Here's how the part is built. I have some questions about the finished solid (model axes, mm). Face numbers are marked on the shaded views. A direction names the side the tool comes from. Coordinates: 2 decimals unless noted, no trailing zeros. Write each loop counter-clockwise with the first axis right and the second up, starting at its lowest first coordinate (ties: lowest second). Pieces come first, ordered by that corner, then holes.
```python
from build123d import *

# Parameters (mm, degrees)
SKETCH1_W           = 84.836
SKETCH1_H           = 69.342
BASE_FLANGE1_DEPTH  = 4.826
SKETCH6_R           = 2.54
CUT_EXTRUDE1_DEPTH  = 10
FILLET1_R           = 2.6
SKETCH7_W           = 18.5
SKETCH7_H           = 10
SKETCH7_W_2         = 39.8249902
SKETCH7_H_2         = 5
CUT_EXTRUDE2_DEPTH  = 4.826
FILLET2_R           = 2.4
FILLET3_R           = 1.6
SKETCH11_W          = 4.445
SKETCH11_H          = 18.2239968
SKETCH11_H_2        = 48.82401137
SKETCH11_W_2        = 50.8
SKETCH11_H_3        = 4.445
BOSS_EXTRUDE1_DEPTH = 24.638


# Sheet-metal steps are written as plain solids
with BuildPart() as part:
    # Sketch1 → Base-Flange1 (new body)
    with BuildSketch(Plane.XY):
        Rectangle(SKETCH1_W, SKETCH1_H)
    extrude(amount=-BASE_FLANGE1_DEPTH)

    # Sketch6 → Cut-Extrude1 (cut)
    with BuildSketch(Plane.XY):
        with Locations((-37.465, 29.718)):
            Circle(SKETCH6_R)
        with Locations(Location((-37.465, -29.718, 0), (0, 0, 180))):
            Circle(SKETCH6_R)
        with Locations((37.465, -29.718)):
            Circle(SKETCH6_R)
        with Locations(Location((37.465, 29.718, 0), (0, 0, 180))):
            Circle(SKETCH6_R)
    extrude(amount=-CUT_EXTRUDE1_DEPTH, mode=Mode.SUBTRACT)

    # Fillet1
    fillet1_edges = [part.edges().sort_by_distance(p)[0] for p in [
        (-42.418, 34.671, -2.413),
        (42.418, 34.671, -2.413),
        (42.418, -34.671, -2.413),
        (-42.418, -34.671, -2.413),
    ]]
    fillet(fillet1_edges, radius=FILLET1_R)

    # Sketch7 → Cut-Extrude2 (cut)
    with BuildSketch(Plane.XY):
        with Locations((-33.168, 18.7119922)):
            Rectangle(SKETCH7_W, SKETCH7_H)
        Polygon((-42.418, -4.5120046), (-27.432, -4.5120046), (-27.432, -26.512012), (-35.052, -26.512012), (-35.052, -17.5120046), (-42.418, -17.5120046), align=None)
        with Locations((7.7044931, 24.3120114)):
            Rectangle(SKETCH7_W_2, SKETCH7_H_2)
        Polygon((-14.2080054, -21.81200997), (-14.2080054, -1.41199997), (-23.2080054, -1.41199997), (-23.2080054, -26.81199997), (27.6169882, -26.81199997), (27.6169882, -21.81200997), align=None)
        Polygon((24.638, 3.195999958), (-11.43, 3.195999958), (-11.43, 15.895999958), (29.21, 15.895999958), (29.21, 3.195999958), (29.21, -6.804000042), (24.638, -6.804000042), align=None)
    extrude(amount=-CUT_EXTRUDE2_DEPTH, mode=Mode.SUBTRACT)

    # Fillet2
    fillet2_edges = [part.edges().sort_by_distance(p)[0] for p in [
        (-12.208002, 21.8120114, -2.413),
        (-12.208002, 26.8120114, -2.413),
        (27.6169882, 26.8120114, -2.413),
        (27.6169882, 21.8120114, -2.413),
        (27.6169882, -21.81200997, -2.413),
        (27.6169882, -26.81199997, -2.413),
        (-23.2080054, -26.81199997, -2.413),
        (-14.2080054, -21.81200997, -2.413),
        (24.638, 3.195999958, -2.413),
        (-27.432, -26.512012, -2.413),
        (-35.052, -26.512012, -2.413),
    ]]
    fillet(fillet2_edges, radius=FILLET2_R)

    # Fillet3
    fillet3_edges = [part.edges().sort_by_distance(p)[0] for p in [
        (-23.2080054, -1.41199997, -2.413),
        (-14.2080054, -1.41199997, -2.413),
        (24.638, -6.804000042, -2.413),
        (-11.43, 3.195999958, -2.413),
        (-11.43, 15.895999958, -2.413),
        (29.21, 15.895999958, -2.413),
        (29.21, -6.804000042, -2.413),
        (-23.918, 23.7119922, -2.413),
        (-23.918, 13.7119922, -2.413),
        (-27.432, -4.5120046, -2.413),
    ]]
    fillet(fillet3_edges, radius=FILLET3_R)

    # Sketch11 → Boss-Extrude1 (add)
    with BuildSketch(Plane(origin=(0, 0, -4.826), x_dir=(-1, 0, 0), z_dir=(0, 0, -1))):
        with Locations((40.1955, 4.5999938)):
            Rectangle(SKETCH11_W, SKETCH11_H)
        with Locations((-40.1955, 5.715e-06)):
            Rectangle(SKETCH11_W, SKETCH11_H_2)
        with Locations((-0.463533105, -32.4485)):
            Rectangle(SKETCH11_W_2, SKETCH11_H_3)
        with Locations((-0.463533105, 32.4485)):
            Rectangle(SKETCH11_W_2, SKETCH11_H_3)
    extrude(amount=BOSS_EXTRUDE1_DEPTH)


solid = part.part
```
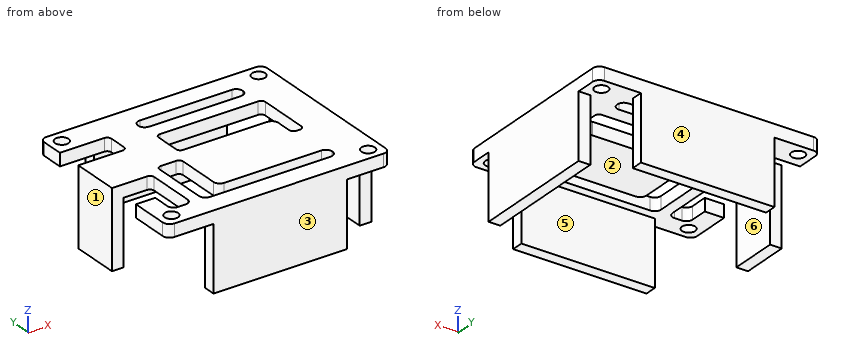
1) I need wall thicknesses on probe 1 along Y at (x, z) = (-6, -0.75); probe 2 along X at (y, z) = (10, -7.25); probe 3 along Y at (x, z) = (-12.5, -25.25). Which ranges of each line are inside material? Lowest first, please.
Values follow:
probe 1: y = -34.67 to -26.81, -21.81 to 3.2, 15.9 to 21.81, 26.81 to 34.67
probe 2: x = -42.42 to -37.97, 37.97 to 42.42
probe 3: y = -34.67 to -30.23, 30.23 to 34.67
2) Imagine slicing it at A-A on z = -12. Please give me the cut outline in (x, y).
Values follow:
outline: (-42.42, -4.51) - (-37.97, -4.51) - (-37.97, 13.71) - (-42.42, 13.71) - close; (-24.94, -34.67) - (25.86, -34.67) - (25.86, -30.23) - (-24.94, -30.23) - close; (-24.94, 30.23) - (25.86, 30.23) - (25.86, 34.67) - (-24.94, 34.67) - close; (37.97, -24.41) - (42.42, -24.41) - (42.42, 24.41) - (37.97, 24.41) - close
3) We'd pull the mould along X, two halves only. Please class the marked faces 1, 2 and 3: pulls with the +X half, pulls with the -X half, needs draft (parallel to the pull), parting line crosses it, or undercut.
Values follow:
face 1: pulls with the -X half
face 2: undercut
face 3: needs draft
4) Will these pins go through, and if not, where does the flat tip stop? pin 1 (4 mm diameter, centred on x = 26.5, z = -9.5, fed in from +Y); pin 2 (1.3 mm diameter, centred on x = 41, z = -18.5, fed in from +Y); pin 3 (1 mm diameter, centred on x = 28, y = -3, fed in from -Z); pin 4 (1.4 mm diameter, centred on y = -12.5, z = -2, fed in from -X).
Values follow:
pin 1: stops at y = 34.67
pin 2: stops at y = 24.41
pin 3: passes through
pin 4: stops at x = -27.43
5) Imagine slicing it at B-B on y = -9. Please give me the cut outline in (x, z).
Values follow:
outline: (-27.43, -4.83) - (-23.21, -4.83) - (-23.21, 0) - (-27.43, 0) - close; (-14.21, -4.83) - (37.97, -4.83) - (37.97, -29.46) - (42.42, -29.46) - (42.42, 0) - (-14.21, 0) - close
6) Imagine slicing it at C-C on y = -23. Please give me the cut outline in (x, z).
Values follow:
outline: (-42.42, -4.83) - (-35.05, -4.83) - (-35.05, 0) - (-42.42, 0) - close; (-27.43, -4.83) - (-23.21, -4.83) - (-23.21, 0) - (-27.43, 0) - close; (27.29, -4.83) - (37.97, -4.83) - (37.97, -29.46) - (42.42, -29.46) - (42.42, 0) - (27.29, 0) - close
7) Imagine slicing it at D-D on x = -36. Please give me the cut outline in (y, z).
Values follow:
outline: (-34.67, -4.83) - (-31.79, -4.83) - (-31.79, 0) - (-34.67, 0) - close; (-27.64, -4.83) - (-17.51, -4.83) - (-17.51, 0) - (-27.64, 0) - close; (-4.51, -4.83) - (13.71, -4.83) - (13.71, 0) - (-4.51, 0) - close; (23.71, -4.83) - (27.64, -4.83) - (27.64, 0) - (23.71, 0) - close; (31.79, -4.83) - (34.67, -4.83) - (34.67, 0) - (31.79, 0) - close
8) On a 3-axis mill with a long thin cutter (end or side, diameter ignored), from which of +Z, -Z, +X, -X, +Y, -Y can I reach the whole of each face in a straight line? I mean the marked faces 4, 5 and 6. Say none if no direction works.
Values follow:
face 4: +Z, -Z, +X, -X, +Y
face 5: -Z, +X, -X
face 6: -Z, +Y, -Y
